Autodesk Inventor part; units mm, degrees
ref_plane "YZ Plane" through (0, 0, 0) normal (1, 0, 0) x (0, 1, 0)
ref_plane "XZ Plane" through (0, 0, 0) normal (0, 1, 0) x (-1, 0, 0)
ref_plane "XY Plane" through (0, 0, 0) normal (0, 0, 1) x (1, 0, 0)
sketch "Sketch1" plane through (0, 0, 0) normal (0, 0, 1) x (1, 0, 0)
  circle A0 centre (0, 0) radius 447.675
  circle A1 centre (0, 0) radius 319.0875
  dimension "d0" = 895.35
  dimension "d1" = 638.175
extrude "Extrusion1" add sketch "Sketch1" along normal blind 3.175
sketch "Sketch2" plane through (0, 0, 3.175) normal (0, 0, 1) x (1, 0, 0)
  circle A0 centre (0, 0) radius 319.0875
  circle A1 centre (0, 0) radius 447.675
  circle A2 centre (342.9, 0) radius 7.1437
  circle A3 centre (419.1, 0) radius 7.9375
  dimension "d4" = 14.2875
  dimension "d5" = 15.875
  dimension "d6" = 342.9
  dimension "d7" = 0
  dimension "d10" = 0
  dimension "d11" = 419.1
extrude "Extrusion2" cut sketch "Sketch2" against normal blind 3.175 contours A2 | A3
pattern_circular "Circular Pattern1" count 16 over 360 about axis through (0, 0, 0) along (0, 0, 1) of "Extrusion2"
properties part number "cover plate" material "Steel, Mild"
Check sheet for the modelled part. Datum: model origin and axes. Units: mm. Round coordinates to 2 decimals unless told otherwise and drop trailing zeros. Order: outer loops, then holes, each group sorted by start corner. A loop starts at its lowest first (then second) coordinate and runs counter-clockwise, first axis right, second up.
Q1. Draft check along Y on faces 1 (the face through (-2, -330, 0)), 2 (the face through (427, -134.47, 1.57)), 3 (the face through (304.35, -95.85, 1.57)). Enter one of: pulls with the +Y half, pulls with the -Y half, needs draft (parallel to the pull), parting line crosses it, or undercut.
Filled sheet:
face 1: needs draft
face 2: parting line crosses it
face 3: undercut
Q2. Cross-section at B-B, the plane x = -69.5. Enter the section's corners in (y, z) (3 decimals).
Filled sheet:
outline: (-442.247, 0) - (-311.427, 0) - (-311.427, 3.175) - (-442.247, 3.175) - close; (311.427, 0) - (442.247, 0) - (442.247, 3.175) - (311.427, 3.175) - close
Q3. Cross-section at A-A, the plane y = 29. Enter the section's corners in (x, z) (3 decimals).
Filled sheet:
outline: (-446.735, 0) - (-317.767, 0) - (-317.767, 3.175) - (-446.735, 3.175) - close; (317.767, 0) - (446.735, 0) - (446.735, 3.175) - (317.767, 3.175) - close
Q4. Scan lines: L1, parallel to X at y = 388, z = 0.8; L2, parallel to X at y = 245.5, z = 2.6. Record each from-to range of solid material in increasing order.
Filled sheet:
L1: x = -223.31 to -168.28, -152.49 to 152.49, 168.28 to 223.31
L2: x = -374.36 to -248.93, -236 to -203.83, 203.83 to 236, 248.93 to 374.36
